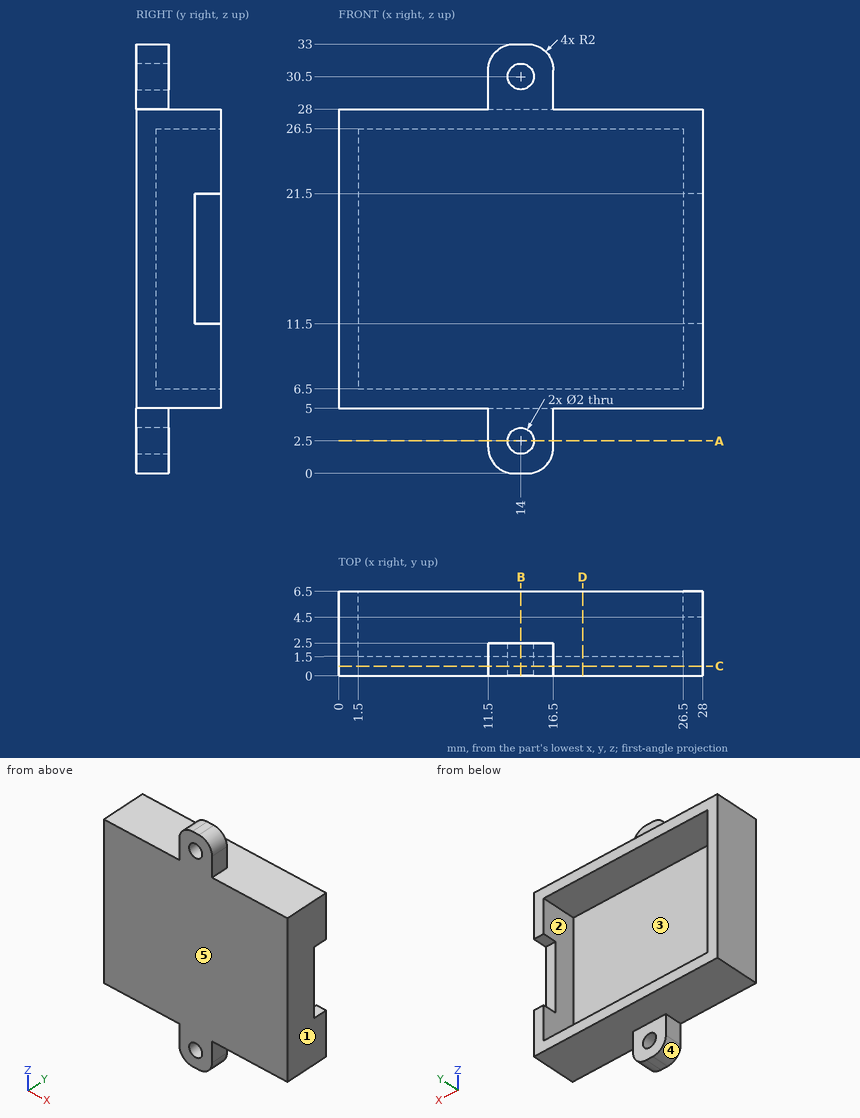
Design review of the part shown in the three views and the two pictorial views. Dimensions are in mm from the part's minimum x, y and z. A direction names the side the tool comes from. Give positions to 0.01 mm unless a question says otherwise; leave off trailing zeros. Loops run counter-clockwise (first coordinate to the right, second up) from the corner with the lowest first, then second, coordinate; pieces in that order, holes last. Notation, with made-up numbers: (15.25, 12) -> (71.25, 12) arc R23 cw to (71.25, 34) -> close; hole circle Ø4 at (-37, 13.5). An arc over 180 degrees is marked (long way). Write each question's results on one line, items separated by ' | '.
Q1. Wall thickness on L1, parallel to X at y = 0.8, z = 30.5; L2, parallel to X at y = 5, z = 22; L3, parallel to Z at x = 13.5, y = 0.75: over which ranges is each line inside the solid? List them lowest first.
Reply:
L1: x = 11.5 to 13, 15 to 16.5 | L2: x = 0 to 1.5, 26.5 to 28 | L3: z = 0 to 1.63, 3.37 to 29.63, 31.37 to 33
Q2. Take a section at D-D, the plane x = 18.75. Write out the cut boundary in (y, z).
Reply:
outline: (0, 5) -> (6.5, 5) -> (6.5, 6.5) -> (1.5, 6.5) -> (1.5, 26.5) -> (6.5, 26.5) -> (6.5, 28) -> (0, 28) -> close
Q3. The part is to be moulded in two halves that separate along Z. For the marked faces 3, 4 and 5, say which applies: +Z half, -Z half, draft (parallel to the pull), parting line (faces both ways), or undercut.
Reply:
face 3: undercut | face 4: -Z half | face 5: draft
Q4. Take a section at A-A, the plane z = 2.5. Write out the cut boundary in (x, y).
Reply:
outline: (11.5, 0) -> (13, 0) -> (13, 2.5) -> (11.5, 2.5) -> close; (15, 0) -> (16.5, 0) -> (16.5, 2.5) -> (15, 2.5) -> close
Q5. Take a section at B-B, the plane x = 14. Write out the cut boundary in (y, z), plus the area to 3 significant figures.
Reply:
outline: (0, 0) -> (2.5, 0) -> (2.5, 1.5) -> (0, 1.5) -> close; (0, 3.5) -> (2.5, 3.5) -> (2.5, 5) -> (6.5, 5) -> (6.5, 6.5) -> (1.5, 6.5) -> (1.5, 26.5) -> (6.5, 26.5) -> (6.5, 28) -> (2.5, 28) -> (2.5, 29.5) -> (0, 29.5) -> close; (0, 31.5) -> (2.5, 31.5) -> (2.5, 33) -> (0, 33) -> close | area: 64.5 mm²
Q6. For pin 1 Ø4 at (x, z) = (13.5, 1.5) entering from +Y; pin 2 Ø2 at (x, z) = (18, 23.5) entering from +Y; pin 3 Ø1.6 at (x, z) = (14, 30.5) entering from +Y; pin 4 Ø1.5 at (x, y) = (19, 3) entering from +Z, all flat-tipped, find the tip position at first contact; note any pin that passes through.
Reply:
pin 1: stops at y = 2.5 | pin 2: stops at y = 1.5 | pin 3: passes through | pin 4: stops at z = 28
Q7. Machinability: for the marked faces 1 and 2, which of the approach directions +Z, -Z, +X, -X, +Y, -Y give a long, thin tool a straight path to every point of the face, cutting with its end or side? Answer none if there is none.
Reply:
face 1: +Z, -Z, +X, +Y, -Y | face 2: +Y
Q8. Take a section at C-C, the plane y = 0.75. Write out the cut boundary in (x, z).
Reply:
outline: (0, 5) -> (11.5, 5) -> (11.5, 2) arc R2 ccw to (13.5, 0) -> (14.5, 0) arc R2 ccw to (16.5, 2) -> (16.5, 5) -> (28, 5) -> (28, 28) -> (16.5, 28) -> (16.5, 31) arc R2 ccw to (14.5, 33) -> (13.5, 33) arc R2 ccw to (11.5, 31) -> (11.5, 28) -> (0, 28) -> close; hole circle Ø2 at (14, 2.5); hole circle Ø2 at (14, 30.5)
